Could you check a few things on this model? Use its own coordinates, in mm. Face numbers are marked on the shaded views. A direction names the side the tool comes from. Give positions to 0.01 mm unless a question says otherwise; leave off trailing zeros. Loops run counter-clockwise (first coordinate to the right, second up) from the corner with the lowest first, then second, coordinate; pieces in that order, holes last. Notation, with made-up numbers: M -6,-6 L 18,-6 A10 ccw 18,0 Z; hole C 6,-35.75 d7. An arc over 180 degrees is marked long. Use a Markdown table: item, result. Add a question column.
1) Suppose I cut it at B-B on y = 0. List the corners of the cut face in (x, z) for me.
2) Suppose I cut it at C-C on x = 1.75. List the corners of the cut face in (y, z) for me.
3) Will these pins go through, and if not, where does the flat tip stop? pin 1 Ø8 at (x, y) = (-7.5, -6.5) entering from -Z; pin 2 Ø1 at (y, z) = (-8.5, 19.5) entering from -X; pin 3 Ø3 at (x, y) = (-1, -12.5) entering from -Z; pin 4 Ø3.5 at (y, z) = (-15, 10) entering from -X.
4) Suppose I cut it at D-D on y = 6.75. List the corners of the cut face in (x, z) for me, and give its area (3 significant figures).
5) If I drill on line 1 along X through (y, z) = (-2, 50); line 2 along Z through (x, y) = (-6.25, 3.75); line 3 along Z through (x, y) = (3.25, 3.75), over which ranges is the centre line in solid material (lowest first)? Write a range as [from, to].
6) Suppose I cut it at A-A on z = 11.5. List the corners of the cut face in (x, y) for me.
7) Which directions (+Z, -Z, +X, -X, +Y, -Y) give clear straight access to the entire face, cutting with the end or side of a thin tool? Please do the marked faces 1, 2, 3, 4 and 5.
```python
from build123d import *
from build123d.topology import SkipClean

# Parameters (mm, degrees)
SKETCH2_R               = 11
BOSS_EXTRUDE1_DEPTH     = 20
BOSS_EXTRUDE2_DEPTH     = 50
BOSS_EXTRUDE3_START     = -50
BOSS_EXTRUDE3_DEPTH     = 5
CUT_EXTRUDE2_DEPTH      = 72.992538676
CUT_EXTRUDE2_DEPTH_BACK = 72.992538676
SKETCH5_R               = 16.440704867
SKETCH5_R_2             = 12.7
BOSS_EXTRUDE4_START     = -5
BOSS_EXTRUDE4_DEPTH     = 30
CUT_EXTRUDE3_START      = 5
SKETCH7_W               = 3.75
SKETCH7_H               = 16.575715954
CUT_EXTRUDE3_DEPTH      = 25


with BuildPart() as part:
    # Sketch2 → Boss-Extrude1 (new body)
    with BuildSketch(Plane.XY):
        Circle(SKETCH2_R)
    extrude(amount=BOSS_EXTRUDE1_DEPTH)

    # Sketch3 → Boss-Extrude2 (add)
    with SkipClean():  # the faces are left unmerged after this step: merging them gives an invalid solid
        with BuildSketch(Plane.XY.offset(20)):
            with BuildLine():
                Line((3.75, 10.34105894), (3.75, -10.34105894))
                ThreePointArc((3.75, -10.34105894), (0, -11), (-3.75, -10.34105894))
                Line((-3.75, -10.34105894), (-3.75, 10.34105894))
                ThreePointArc((-3.75, 10.34105894), (0, 11), (3.75, 10.34105894))
            make_face()
        extrude(amount=BOSS_EXTRUDE2_DEPTH)

    # Sketch4 → Boss-Extrude3 (add)
    with SkipClean():  # the faces are left unmerged after this step: merging them gives an invalid solid
        with BuildSketch(Plane.XY.offset(70).offset(BOSS_EXTRUDE3_START)):
            with BuildLine():
                Line((-3.75, -10.34105894), (-3.75, -12.159898231))
                ThreePointArc((-3.75, -12.159898231), (0, -12.725), (3.75, -12.159898231))
                Line((3.75, -12.159898231), (3.75, -10.34105894))
                ThreePointArc((3.75, -10.34105894), (0, -11), (-3.75, -10.34105894))
            make_face()
        extrude(amount=BOSS_EXTRUDE3_DEPTH)

    # Sketch5 → Cut-Extrude2 (cut, two sides: drawn at the far end of the back side and taken through both)
    with SkipClean():  # the faces are left unmerged after this step: merging them gives an invalid solid
        with BuildSketch(Plane.XY.offset(70).offset(-CUT_EXTRUDE2_DEPTH_BACK)):
            Circle(SKETCH5_R)
            Circle(SKETCH5_R_2, mode=Mode.SUBTRACT)
        extrude(amount=CUT_EXTRUDE2_DEPTH + CUT_EXTRUDE2_DEPTH_BACK, mode=Mode.SUBTRACT)

    # Sketch6 → Boss-Extrude4 (add)
    with SkipClean():  # the faces are left unmerged after this step: merging them gives an invalid solid
        with BuildSketch(Plane(origin=(0, 0, 20), x_dir=(-1, 0, 0), z_dir=(0, 0, -1)).offset(BOSS_EXTRUDE4_START)):
            with BuildLine():
                Line((-3.75, -12.133733968), (-3.75, -15.55434023))
                ThreePointArc((-3.75, -15.55434023), (0, -16), (3.75, -15.55434023))
                Line((3.75, -15.55434023), (3.75, -12.133733968))
                ThreePointArc((3.75, -12.133733968), (0, -12.7), (-3.75, -12.133733968))
            make_face()
        extrude(amount=BOSS_EXTRUDE4_DEPTH)

    # Sketch7 → Cut-Extrude3 (cut)
    with SkipClean():  # the faces are left unmerged after this step: merging them gives an invalid solid
        with BuildSketch(Plane(origin=(0, 0, 0), x_dir=(-1, 0, 0), z_dir=(0, 0, -1)).offset(CUT_EXTRUDE3_START)):
            with Locations((1.875, -20.421591945)):
                Rectangle(SKETCH7_W, SKETCH7_H)
        extrude(amount=-CUT_EXTRUDE3_DEPTH, mode=Mode.SUBTRACT)


solid = part.part
```
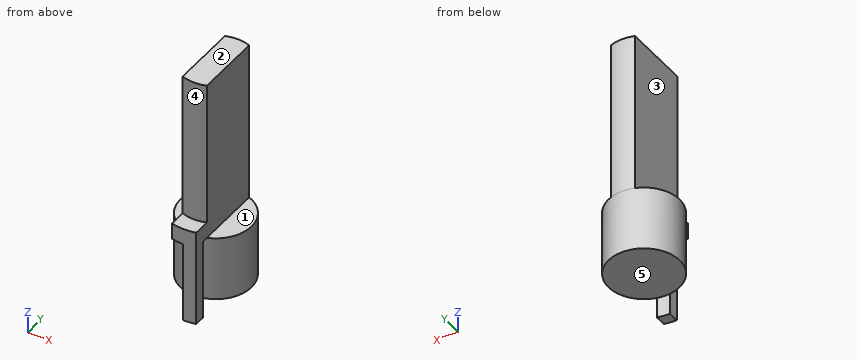
Answer block:
| question | item | result |
|---|---|---|
| 1 | outline | M -11,0 L 11,0 L 11,20 L 3.75,20 L 3.75,70 L -3.75,70 L -3.75,20 L -11,20 Z |
| 2 | outline | M -15.9,-5 L -12.58,-5 L -12.58,20 L -10.86,20 L -10.86,0 L 10.86,0 L 10.86,70 L -10.86,70 L -10.86,25 L -15.9,25 Z |
| 3 | pin 1 | stops at z = 0 |
| 3 | pin 2 | stops at x = -7.55 |
| 3 | pin 3 | stops at z = -5 |
| 3 | pin 4 | stops at x = 0 |
| 4 | outline | M -8.69,0 L 8.69,0 L 8.69,20 L 3.75,20 L 3.75,70 L -3.75,70 L -3.75,20 L -8.69,20 Z |
| 4 | area | 722 mm^2 |
| 5 | line 1 | x = [-3.75, 3.75] |
| 5 | line 2 | z = [0, 20] |
| 5 | line 3 | z = [0, 70] |
| 6 | outline | C 0,0 d22; M 0,-16 A16 ccw 3.75,-15.55 L 3.75,-12.13 A12.7 cw 0,-12.7 Z |
| 7 | face 1 | +Z, +X, +Y, -Y |
| 7 | face 2 | +Z, +X, -X, +Y, -Y |
| 7 | face 3 | +Z, -X, +Y, -Y |
| 7 | face 4 | +Z, -Y |
| 7 | face 5 | -Z, +X, -X, +Y |
